from build123d import *

# Parameters (mm, degrees)
SKETCH1_W           = 100
SKETCH1_H           = 41
BOSS_EXTRUDE1_DEPTH = 42.1
SKETCH2_R           = 4.5
CUT_EXTRUDE1_DEPTH  = 41
SKETCH1_3_R         = 4.5
BOSS_EXTRUDE2_DEPTH = 10


with BuildPart() as part:
    # Sketch1 → Boss-Extrude1 (new body)
    with BuildSketch(Plane.XY):
        with Locations((50, -20.5)):
            Rectangle(SKETCH1_W, SKETCH1_H)
        Polygon((79.207902433, -4.44375), (72.792097567, -4.44375), (69.584195134, -10), (72.792097567, -15.55625), (79.207902433, -15.55625), (82.415804866, -10), align=None, mode=Mode.SUBTRACT)
        Polygon((20.792097567, -15.55625), (17.584195134, -10), (20.792097567, -4.44375), (27.207902433, -4.44375), (30.415804866, -10), (27.207902433, -15.55625), align=None, mode=Mode.SUBTRACT)
    extrude(amount=BOSS_EXTRUDE1_DEPTH)

    # Sketch2 → Cut-Extrude1 (cut)
    with BuildSketch(Plane(origin=(0, 0, 0), x_dir=(-1, 0, 0), z_dir=(0, -1, 0))):
        with Locations(Location((-10, -23, 0), (0, 0, 270))):
            Circle(SKETCH2_R)
        with Locations(Location((-50, -23, 0), (0, 0, 270))):
            Circle(SKETCH2_R)
        with Locations(Location((-90, -23, 0), (0, 0, 270))):
            Circle(SKETCH2_R)
    extrude(amount=CUT_EXTRUDE1_DEPTH, mode=Mode.SUBTRACT)

    # Sketch1<3> → Boss-Extrude2 (add)
    # profile 1 of 2: a face of its own
    with BuildSketch(Plane.XY):
        Polygon((27.207902433, -4.44375), (20.792097567, -4.44375), (17.584195134, -10), (20.792097567, -15.55625), (27.207902433, -15.55625), (30.415804866, -10), align=None)
        with Locations((24, -10)):
            Circle(SKETCH1_3_R, mode=Mode.SUBTRACT)
    # profile 2 of 2: a face of its own
    with BuildSketch(Plane.XY):
        Polygon((79.207902433, -15.55625), (82.415804866, -10), (79.207902433, -4.44375), (72.792097567, -4.44375), (69.584195134, -10), (72.792097567, -15.55625), align=None)
        with Locations((76, -10)):
            Circle(SKETCH1_3_R, mode=Mode.SUBTRACT)
    extrude(amount=BOSS_EXTRUDE2_DEPTH)


solid = part.part
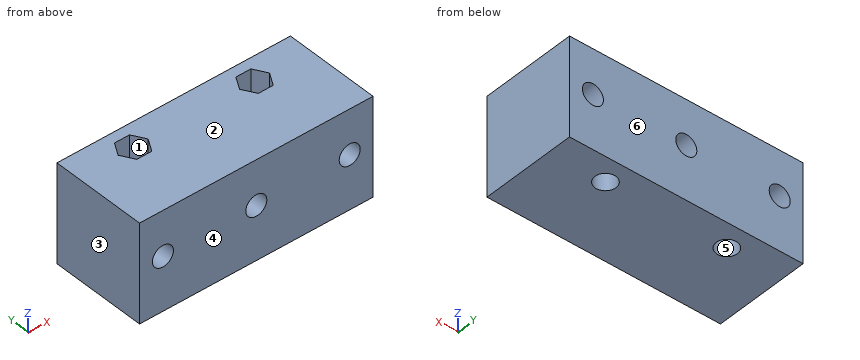
Design review of the part built by this model. Coordinates are the model's own, in mm. Face numbers are marked on the shaded views. A direction names the side the tool comes from. Give positions to 0.01 mm unless a question says otherwise; leave off trailing zeros. Order: outer loops, then holes, each group sorted by start corner. A loop starts at its lowest first (then second) coordinate and runs counter-clockwise, first axis right, second up.
1. To check wall thickness, follow L1, parallel to X at y = -29, z = 23; L2, parallel to Z at x = 50, y = -19; L3, parallel to Y at x = 27, z = 27.5. State the ranges of each line that lie inside material, in increasing order.
Solution:
L1: x = 0 to 5.5, 14.5 to 45.5, 54.5 to 85.5, 94.5 to 100
L2: z = 0 to 18.5, 27.5 to 42.1
L3: y = -41 to -15.56, -4.44 to 0
2. Add section A-A, the plane z = 23. State the section outline as (x, y) points, then the cut area to 3 significant figures.
Solution:
outline: (0, -41) - (5.5, -41) - (5.5, 0) - (0, 0) - close; (14.5, -41) - (45.5, -41) - (45.5, 0) - (14.5, 0) - close; (54.5, -41) - (85.5, -41) - (85.5, 0) - (54.5, 0) - close; (94.5, -41) - (100, -41) - (100, 0) - (94.5, 0) - close; hole (17.58, -10) - (20.79, -15.56) - (27.21, -15.56) - (30.42, -10) - (27.21, -4.44) - (20.79, -4.44) - close; hole (69.58, -10) - (72.79, -15.56) - (79.21, -15.56) - (82.42, -10) - (79.21, -4.44) - (72.79, -4.44) - close
area: 2,780 mm2
3. Mouldability with a two-part tool opening along Y and no side actions: class the marked faces 3, 4, 5 and 6 as +Y half, -Y half, draft (parallel to the pull), parting line (faces both ways), or undercut.
Solution:
face 3: draft
face 4: -Y half
face 5: undercut
face 6: +Y half
4. Add section B-B, the plane x = 24. State the section outline as (y, z) points.
Solution:
outline: (-41, 0) - (-14.5, 0) - (-14.5, 10) - (-15.56, 10) - (-15.56, 42.1) - (-41, 42.1) - close; (-5.5, 0) - (0, 0) - (0, 42.1) - (-4.44, 42.1) - (-4.44, 10) - (-5.5, 10) - close
5. Add section D-D, the plane z = 33. State the section outline as (x, y) points.
Solution:
outline: (0, -41) - (100, -41) - (100, 0) - (0, 0) - close; hole (17.58, -10) - (20.79, -15.56) - (27.21, -15.56) - (30.42, -10) - (27.21, -4.44) - (20.79, -4.44) - close; hole (69.58, -10) - (72.79, -15.56) - (79.21, -15.56) - (82.42, -10) - (79.21, -4.44) - (72.79, -4.44) - close
6. Add section C-C, the plane y = -26.5. State the section outline as (x, z) points.
Solution:
outline: (0, 0) - (100, 0) - (100, 42.1) - (0, 42.1) - close; hole circle Ø9 at (10, 23); hole circle Ø9 at (50, 23); hole circle Ø9 at (90, 23)
7. Tool access review of the marked faces 1 and 2: name each direction out of +Z, -Z, +X, -X, +Y, -Y from which nothing blocks a thin tool from reaching the whole face with its end or side.
Solution:
face 1: +Z
face 2: +Z, +X, -X, +Y, -Y
8. For pin 1 Ø11.5 at (x, z) = (90, 23) entering from -Y, flat-tipped, find the tip position at first contact; note if it passes through.
Solution:
pin 1: stops at y = -41
